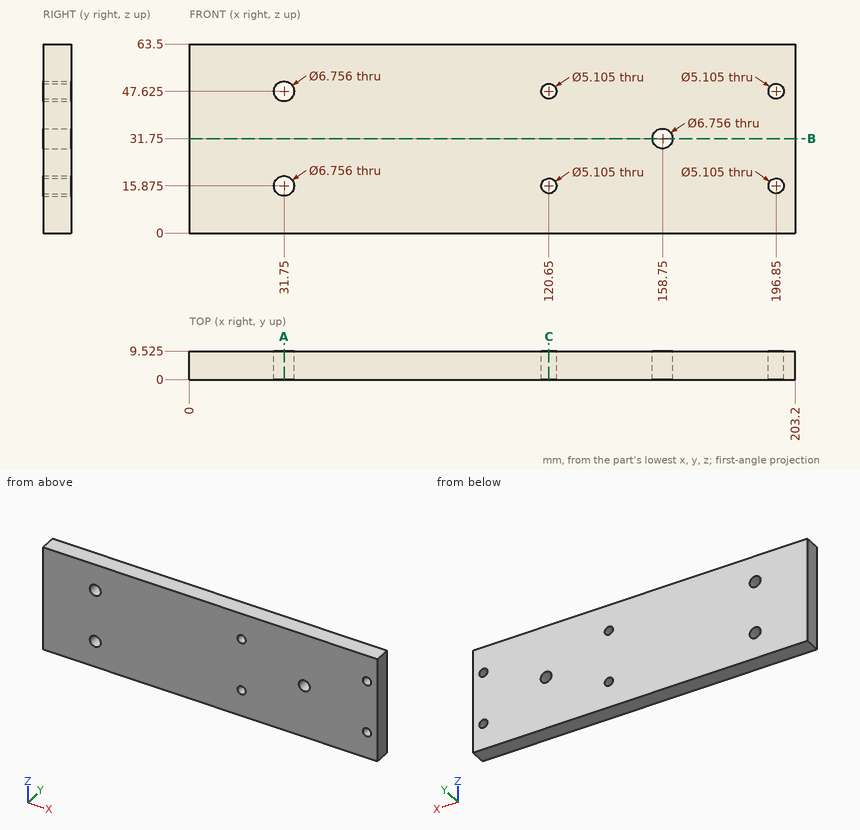
Part print with two shaded views. Sizes in mm from the minimum x, y, z corner. Give positions to 0.01 mm unless a question says otherwise; leave off trailing zeros. Loops run counter-clockwise (first coordinate to the right, second up) from the corner with the lowest first, then second, coordinate; pieces in that order, holes last. Notation, with made-up numbers: (33.25, 31.5) - (75.25, 31.5) arc R37 cw to (75.25, 69.5) - close; hole circle Ø7 at (85.5, -17.75). An arc over 180 degrees is marked (long way). Put each result on its own line as item: value.
Q1. Slice it at A-A (x = 31.75). Give the cut face in (y, z) (1 decimal).
Filled in:
outline: (0, 0) - (9.5, 0) - (9.5, 12.5) - (0, 12.5) - close; (0, 19.3) - (9.5, 19.3) - (9.5, 44.2) - (0, 44.2) - close; (0, 51) - (9.5, 51) - (9.5, 63.5) - (0, 63.5) - close
Q2. Probe line 1 along Z through (x, y) = (31.75, 6); line 2 along Z through (x, y) = (196.85, 4); line 3 along X through (y, z) = (5, 31.75). List the from-to ranges inside material, lowest first.
Filled in:
line 1: z = 0 to 12.5, 19.25 to 44.25, 51 to 63.5
line 2: z = 0 to 13.32, 18.43 to 45.07, 50.18 to 63.5
line 3: x = 0 to 155.37, 162.13 to 203.2
Q3. Slice it at B-B (z = 31.75). Give the cut face in (x, y) (1 decimal), plus the area to 3 significant figures.
Filled in:
outline: (0, 0) - (155.4, 0) - (155.4, 9.5) - (0, 9.5) - close; (162.1, 0) - (203.2, 0) - (203.2, 9.5) - (162.1, 9.5) - close
area: 1,870 mm²
Q4. Slice it at C-C (x = 120.65). Give the cut face in (y, z) (1 decimal).
Filled in:
outline: (0, 0) - (9.5, 0) - (9.5, 13.3) - (0, 13.3) - close; (0, 18.4) - (9.5, 18.4) - (9.5, 45.1) - (0, 45.1) - close; (0, 50.2) - (9.5, 50.2) - (9.5, 63.5) - (0, 63.5) - close
